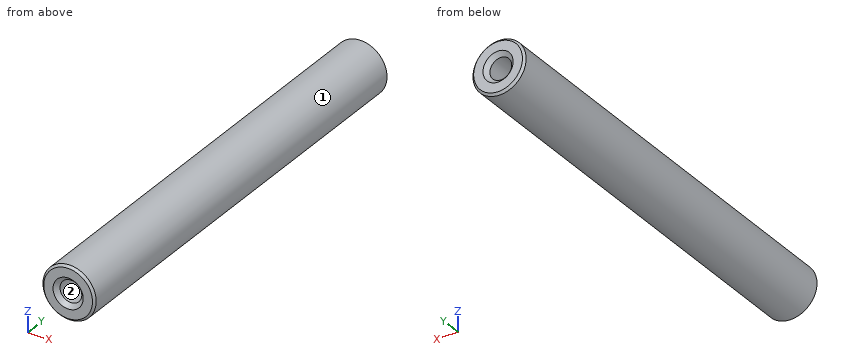
Autodesk Inventor part; units mm, degrees
ref_plane "YZ Plane" through (0, 0, 0) normal (1, 0, 0) x (0, 1, 0)
ref_plane "XZ Plane" through (0, 0, 0) normal (0, 1, 0) x (-1, 0, 0)
ref_plane "XY Plane" through (0, 0, 0) normal (0, 0, 1) x (1, 0, 0)
sketch "スケッチ1" plane through (0, 0, 0) normal (0, 1, 0) x (-1, 0, 0)
  circle A0 centre (0, 0) radius 3
  dimension "d0" = 6
extrude "押し出し1" add sketch "スケッチ1" along normal mid plane 50
sketch "スケッチ2" plane through (0, 25, 0) normal (0, 1, 0) x (1, 0, 0)
  point P0 (0, 0)
  point P1 (0, 0)
hole "穴1" at (0, 25, 0) direction (0, -1, 0) diameter 2.459 depth 10 countersink diameter 3.4 countersink angle 90
sketch "スケッチ3" plane through (0, -25, 0) normal (0, -1, 0) x (1, 0, 0)
  point P0 (0, 0)
  point P1 (0, 0)
hole "穴2" at (0, -25, 0) direction (0, 1, 0) diameter 2.459 depth 10 countersink diameter 3.4 countersink angle 90
chamfer "面取り1" distance 0.25 angle 45 2 edges at (3, -25, 0) (3, 25, 0)
properties part number "Spacer_M3D6L45" material "アルミニウム 6061"
CAD build for the part. Positions are in the model's coordinates, mm. Face numbers are marked on the shaded views. Give positions to 0.01 mm unless a question says otherwise; leave off trailing zeros. Loops run counter-clockwise (first coordinate to the right, second up) from the corner with the lowest first, then second, coordinate; pieces in that order, holes last. Notation, with made-up numbers: (67.25, 37) - (84.25, 37) arc R28 ccw to (84.25, 71) - close; hole circle Ø1 at (78, 68). An arc over 180 degrees is marked (long way). Put each result on its own line as item: value.
Q1. Slice it at A-A (z = 0). Give the cut face in (x, y).
Filled in:
outline: (-3, -24.75) - (-2.75, -25) - (-1.7, -25) - (-1.23, -24.53) - (-1.23, -15) - (1.23, -15) - (1.23, -24.53) - (1.7, -25) - (2.75, -25) - (3, -24.75) - (3, 24.75) - (2.75, 25) - (1.7, 25) - (1.23, 24.53) - (1.23, 15) - (-1.23, 15) - (-1.23, 24.53) - (-1.7, 25) - (-2.75, 25) - (-3, 24.75) - close
Q2. Probe line 1 along Z through (x, y) = (0, 21.75); line 2 along Y through (x, z) = (-0.8, 0.4); line 3 along Z through (x, y) = (1.2, 3). List the from-to ranges inside material, lowest first.
Filled in:
line 1: z = -3 to -1.23, 1.23 to 3
line 2: y = -15 to 15
line 3: z = -2.75 to 2.75
Q3. Mould opens along Z. For the marked faces 1 and 2 say: pulls with the +Z half, pulls with the -Z half, needs draft (parallel to the pull), parting line crosses it, or undercut.
Filled in:
face 1: parting line crosses it
face 2: undercut
Q4. Slice it at C-C (y = -19.5). Give the cut face in (x, z).
Filled in:
outline: circle Ø6 at (0, 0); hole circle Ø2.46 at (0, 0)
Q5. Slice it at B-B (x = 0). Give the cut face in (y, z), plus the area to 3 significant figures.
Filled in:
outline: (-25, -2.75) - (-24.75, -3) - (24.75, -3) - (25, -2.75) - (25, -1.7) - (24.53, -1.23) - (15, -1.23) - (15, 1.23) - (24.53, 1.23) - (25, 1.7) - (25, 2.75) - (24.75, 3) - (-24.75, 3) - (-25, 2.75) - (-25, 1.7) - (-24.53, 1.23) - (-15, 1.23) - (-15, -1.23) - (-24.53, -1.23) - (-25, -1.7) - close
area: 250 mm²
Q6. Slice it at D-D (y = 9). Give the cut face in (x, z), plus the area to 3 significant figures.
Filled in:
outline: circle Ø6 at (0, 0)
area: 28.3 mm²
Q7. Flat gauge pins, fed straight in: pin 1 (3 mm diameter, centred on y = 0, z = -2.5, fed in from +X); pin 2 (3 mm diameter, centred on x = 0, z = 0, fed in from +Y); pin 3 (1.2 mm diameter, centred on x = -0.5, z = -0.5, fed in from -Y). Where does each tip first touch, or does it go through?
Filled in:
pin 1: stops at x = 2.83
pin 2: stops at y = 24.8
pin 3: stops at y = -24.61
